Model file for the job. Use its own axes, mm. Face numbers are marked on the shaded views. A direction names the side the tool comes from. Round coordinates to 2 decimals unless told otherwise and drop trailing zeros. Loops run counter-clockwise (first coordinate to the right, second up) from the corner with the lowest first, then second, coordinate; pieces in that order, holes last.
from build123d import *

# Parameters (mm, degrees)
CUT_EXTRUDE_1_DEPTH = 8
EXTRUDE_START       = 7
SKETCH_3_R          = 2.5
EXTRUDE_1_DEPTH     = 7


# Read off the part's stored shape, not the designer's step: M5 机械螺纹 螺柱1
with BuildPart() as part:
    # Sketch 1 → 旋转1 (revolve)
    with BuildSketch(Plane.XY, mode=Mode.PRIVATE) as revolve_1_sk:
        Polygon((5, 9), (5, -2), (10, -2), (10, 0), (8.5, 0), (8.5, 9), align=None)
    revolve(revolve_1_sk.sketch.rotate(Axis((5, -2, 0), (0, 1, 0)), 90), axis=Axis((5, -2, 0), (0, 1, 0)))

    # Sketch 2 → 切除-拉伸1 (cut)
    with BuildSketch(Plane(origin=(0, 9, 0), x_dir=(1, 0, 0), z_dir=(0, 1, 0))):
        with BuildLine():
            ThreePointArc((7.449489743, 2.5), (5, 3.5), (2.550510257, 2.5))
            Line((2.550510257, 2.5), (7.449489743, 2.5))
        make_face()
        with BuildLine():
            Line((7.449489743, -2.5), (2.550510257, -2.5))
            ThreePointArc((2.550510257, -2.5), (5, -3.5), (7.449489743, -2.5))
        make_face()
    extrude(amount=-CUT_EXTRUDE_1_DEPTH, mode=Mode.SUBTRACT)

    # M5 机械螺纹 螺柱1 outline → M5 机械螺纹 螺柱1 (revolve)
    with BuildSketch(Plane(origin=(5, 0, 0), x_dir=(1, 0, 0), z_dir=(0, 0, 1))):
        Polygon((2.067, 19), (0, 19), (0, 9), (2.5, 9), (2.5, 18.567), align=None)
    revolve(axis=Axis((5, 0, 0), (0, 1, 0)))

    # 草图3 → 凸台-拉伸1 (add)
    with BuildSketch(Plane(origin=(0, 9, 0), x_dir=(1, 0, 0), z_dir=(0, 1, 0)).offset(EXTRUDE_START)):
        with Locations(Location((5, 0, 0), (0, 0, 90))):
            Circle(SKETCH_3_R)
    extrude(amount=-EXTRUDE_1_DEPTH)


solid = part.part
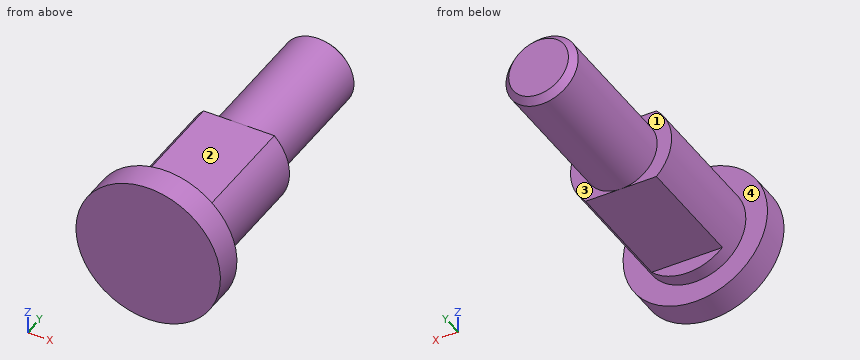
Q1. Slice it at A-A on z = 0. Give the cut face in (x, y), plus the area to 3 significant figures.
Q2. Flat gauge pins, fed straight in: P1, Ø4, axis at x = 4, y = 6.5, coming from the -Z side; P2, Ø4, axis at x = 4.5, y = 5, coming from the +Z side; P3, Ø1.1, axis at x = 5, z = 3, coming from the +Y side. Where does each tip first touch, or does it go through?
Q3. Slice it at C-C on y = 14. Give the cut face in (x, z).
Q4. Probe line 1 (Y direction, x = 3.5, z = 4.25); line 2 (Z direction, x = 4.75, y = 3); line 3 (Y direction, x = 2, z = -0.5). List the from-to ranges inside material, lowest first.
Q5. Slice it at B-B on x = 2. Give the cut face in (y, z).
Q6. Tool access for the marked faces 1, 2, 3 and 4: list every direction of +Z, -Z, +X, -X, +Y, -Y with a clear straight run to the whole face (end or side of a thin tool).
Q7. Slice it at D-D on z = 3.75. Give the cut face in (x, y), plus the area to 3 significant figures.
Reply:
1. outline: (0, -2) - (10, -2) - (10, 0) - (8.5, 0) - (8.5, 9) - (7.5, 9) - (7.5, 18.57) - (7.07, 19) - (2.93, 19) - (2.5, 18.57) - (2.5, 9) - (1.5, 9) - (1.5, 0) - (0, 0) - close
1. area: 133 mm2
2. P1: stops at z = -2.5
2. P2: stops at z = 2.5
2. P3: stops at y = 18.62
3. outline: circle Ø5 at (5, 0)
4. line 1: y = -2 to 0
4. line 2: z = -2.5 to 2.5
4. line 3: y = -2 to 9
5. outline: (-2, -4) - (0, -4) - (0, -1.8) - (9, -1.8) - (9, 1.8) - (0, 1.8) - (0, 4) - (-2, 4) - close
6. face 1: -X, +Y
6. face 2: +Z, +X, -X, +Y
6. face 3: +X, +Y
6. face 4: +Y
7. outline: (1.69, -2) - (8.31, -2) - (8.31, 0) - (1.69, 0) - close
7. area: 13.2 mm2
